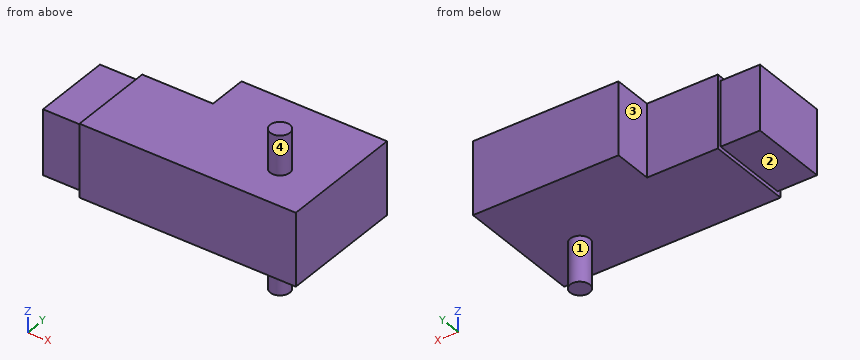
```python
from build123d import *

# Parameters (mm, degrees)
SKETCH1_W                = 55
SKETCH1_H                = 18.5
BOSS_EXTRUDE1_DEPTH      = 22
SKETCH2_W                = 16.5
SKETCH2_H                = 20
BOSS_EXTRUDE2_DEPTH      = 10
BOSS_EXTRUDE3_DEPTH      = 10
BOSS_EXTRUDE3_DEPTH_BACK = 30
SKETCH5_R                = 2.5
SKETCH6_W                = 37
SKETCH6_H                = 18.5
BOSS_EXTRUDE4_DEPTH      = 10


with BuildPart() as part:
    # Sketch1 → Boss-Extrude1 (new body)
    with BuildSketch(Plane(origin=(0, 0, 0), x_dir=(1, 0, 0), z_dir=(0, 1, 0))):
        Rectangle(SKETCH1_W, SKETCH1_H)
    extrude(amount=BOSS_EXTRUDE1_DEPTH)

    # Sketch2 → Boss-Extrude2 (add)
    with BuildSketch(Plane.ZY.offset(27.5)):
        with Locations((0, 11)):
            Rectangle(SKETCH2_W, SKETCH2_H)
    extrude(amount=BOSS_EXTRUDE2_DEPTH)

    # Sketch5 → Boss-Extrude3 (add, two sides: drawn at the far end of the back side and taken through both)
    with BuildSketch(Plane.XY.offset(9.25).offset(-BOSS_EXTRUDE3_DEPTH_BACK)):
        with Locations((15.5, 11.027980953)):
            Circle(SKETCH5_R)
    extrude(amount=BOSS_EXTRUDE3_DEPTH + BOSS_EXTRUDE3_DEPTH_BACK)

    # Sketch6 → Boss-Extrude4 (add)
    with BuildSketch(Plane(origin=(0, 22, 0), x_dir=(1, 0, 0), z_dir=(0, 1, 0))):
        with Locations((9, 0)):
            Rectangle(SKETCH6_W, SKETCH6_H)
    extrude(amount=BOSS_EXTRUDE4_DEPTH)


solid = part.part
```
Could you check a few things on this model? Use its own coordinates, in mm. Face numbers are marked on the shaded views. A direction names the side the tool comes from. Round coordinates to 2 decimals unless told otherwise and drop trailing zeros. Loops run counter-clockwise (first coordinate to the right, second up) from the corner with the lowest first, then second, coordinate; pieces in that order, holes last. Notation, with made-up numbers: M 24.5,-34.75 L 62.5,-34.75 A21 ccw 62.5,-18.75 Z; hole C 0.5,11.25 d7. An arc over 180 degrees is marked long. Write item = value, one per line.
1. I want a section at B-B, the plane z = 2. Write out the boundary of the cut face in (x, y).
Results below:
outline = M -37.5,1 L -27.5,1 L -27.5,0 L 27.5,0 L 27.5,32 L -9.5,32 L -9.5,22 L -27.5,22 L -27.5,21 L -37.5,21 Z
2. Will these pins go through, and if not, where does the flat tip stop? P1, Ø3, axis at x = -32.5, z = 0.5, coming from the -Y side; P2, Ø9.5, axis at x = 1, y = 22.5, coming from the -Z side; P3, Ø5, axis at y = 25, z = -3, coming from the -X side; P4, Ø4, axis at x = -29.5, z = 12, coming from the -Y side (1 decimal).
Results below:
P1 = 1
P2 = -9.25
P3 = -9.5
P4 = through
3. I need wall thicknesses on probe 1 along Z at (x, y) = (10, 30.5); probe 2 along Y at (x, z) = (-31, 1.5); probe 3 along Z at (x, y) = (-29, 8). Which ranges of each line are inside material? Lowest first, please.
Results below:
probe_1 = -9.25 to 9.25
probe_2 = 1 to 21
probe_3 = -8.25 to 8.25
4. I want a section at A-A, the plane y = 3.5. Write out the boundary of the cut face in (x, z).
Results below:
outline = M -37.5,-8.25 L -27.5,-8.25 L -27.5,-9.25 L 27.5,-9.25 L 27.5,9.25 L -27.5,9.25 L -27.5,8.25 L -37.5,8.25 Z
5. Which directions (+Z, -Z, +X, -X, +Y, -Y) give clear straight access to the entire face, cutting with the end or side of a thin tool? Please do the marked faces 1, 2, 3 and 4.
Results below:
face_1 = -Z
face_2 = -Z, -X, +Y, -Y
face_3 = +Z, -Z, -X, +Y
face_4 = +Z
6. I want a section at D-D, the plane y = 28.5. Write out the boundary of the cut face in (x, z).
Results below:
outline = M -9.5,-9.25 L 27.5,-9.25 L 27.5,9.25 L -9.5,9.25 Z
7. I want a section at C-C, the plane x = 15.5. Write out the boundary of the cut face in (y, z).
Results below:
outline = M 0,-9.25 L 8.53,-9.25 L 8.53,-20.75 L 13.53,-20.75 L 13.53,-9.25 L 32,-9.25 L 32,9.25 L 13.53,9.25 L 13.53,19.25 L 8.53,19.25 L 8.53,9.25 L 0,9.25 Z
